```python
from build123d import *

# Parameters (mm, degrees)
EXTRUDE_1_DEPTH           = 18
CHAMFER_1_SIZE            = 5
CHAMFER_2_SIZE            = 5
CUT_EXTRUDE_1_DEPTH       = 8
EXTRUDE_2_REACH           = 696.741
EXTRUDE_2_END_RADIUS      = 240
EXTRUDE_3_DEPTH           = 5
EXTRUDE_4_REACH           = 929.644
EXTRUDE_4_END_RADIUS      = 232
SKETCH_10_R               = 12
CUT_EXTRUDE_7_DEPTH       = 695.872110635
CUT_EXTRUDE_7_DEPTH_BACK  = 695.872110635
SKETCH_16_OUTSIDE_W       = 362.68
SKETCH_16_OUTSIDE_H       = 1204.68
SKETCH_16_OUTSIDE_W_2     = 100
SKETCH_16_OUTSIDE_H_2     = 230
CUT_EXTRUDE_9_DEPTH       = 203.111355445
CUT_EXTRUDE_9_DEPTH_BACK  = 203.111355445
EXTRUDE_5_DEPTH           = 20
CUT_EXTRUDE_10_DEPTH      = 219.63208799
CUT_EXTRUDE_10_DEPTH_BACK = 219.63208799
SKETCH_21_R               = 1.9
EXTRUDE_START             = 15
SKETCH_29_R               = 1.9
EXTRUDE_6_DEPTH           = 15
SKETCH_33_OUTSIDE_W       = 126.318
SKETCH_33_OUTSIDE_H       = 74.662
CUT_EXTRUDE_16_DEPTH      = 40
CUT_EXTRUDE_15_DEPTH      = 41


with BuildPart() as part:
    # Sketch 4 → Loft 1 section 0
    with BuildSketch(Plane(origin=(0, 10, 0), x_dir=(1, 0, 0), z_dir=(0, 1, 0))):
        with BuildLine():
            Line((25, 0), (-25, 0))
            Line((-25, 0), (-25, 630))
            Line((-25, 630), (0, 672.857142857))
            Line((0, 672.857142857), (25, 630))
            Line((25, 630), (25, 0))
        make_face()
    # Sketch 1 → Loft 1 section 1
    with BuildSketch(Plane(origin=(0, 0, 0), x_dir=(1, 0, 0), z_dir=(0, 1, 0))):
        with BuildLine():
            Line((-35, 0), (35, 0))
            Line((35, 0), (35, 630))
            Line((35, 630), (0, 690))
            Line((0, 690), (-35, 630))
            Line((-35, 630), (-35, 0))
        make_face()
    loft_1 = loft()

    # Mirror 1: Loft 1 across plane
    add(loft_1.mirror(Plane.ZX))



with BuildPart() as body_2:
    # Sketch 5 → Extrude 1 (new, symmetric)
    with BuildSketch(Plane(origin=(0, 0, 0), x_dir=(1, 0, 0), z_dir=(0, 1, 0))):
        with BuildLine():
            ThreePointArc((-66.346774613, -65.189169183), (0, -55.5), (66.346774613, -65.189169183))
            ThreePointArc((66.346774613, -65.189169183), (73.061224406, -64.270510235), (76.791165228, -58.612302768))
            ThreePointArc((76.791165228, -58.612302768), (79, -30.5), (76.791165228, -2.387697232))
            ThreePointArc((76.791165228, -2.387697232), (0, -15.004503167), (-76.791165228, -2.387697232))
            ThreePointArc((-76.791165228, -2.387697232), (-79, -30.5), (-76.791165228, -58.612302768))
            ThreePointArc((-76.791165228, -58.612302768), (-73.061224406, -64.270510235), (-66.346774613, -65.189169183))
        make_face()
    extrude(amount=EXTRUDE_1_DEPTH, both=True)

    # Chamfer 1
    chamfer_1_edges = [body_2.edges().sort_by_distance(p)[0] for p in [
        (0, 18, 15.004503167),
        (-79, 18, 30.5),
        (-73.061224406, 18, 64.270510235),
        (0, 18, 55.5),
        (73.061224406, 18, 64.270510235),
        (0, -18, 55.5),
        (-73.061224406, -18, 64.270510235),
        (-79, -18, 30.5),
        (79, -18, 30.5),
        (73.061224406, -18, 64.270510235),
        (79, 18, 30.5),
    ]]
    chamfer(chamfer_1_edges, length=CHAMFER_1_SIZE)

    # Chamfer 2
    chamfer_2_edges = [body_2.edges().sort_by_distance(p)[0] for p in [
        (0, -18, 15.004503167),
    ]]
    chamfer(chamfer_2_edges, length=CHAMFER_2_SIZE)

    # Sketch 6 → Cut-Extrude 1 (cut)
    with BuildSketch(Plane(origin=(0, 18, 0), x_dir=(1, 0, 0), z_dir=(0, 1, 0))):
        with BuildLine():
            ThreePointArc((67.221840199, -55.023712607), (68.932610365, -35.286223394), (68.335500378, -15.483731767))
            ThreePointArc((68.335500378, -15.483731767), (0, -25.004503167), (-68.335500378, -15.483731767))
            ThreePointArc((-68.335500378, -15.483731767), (-68.932610365, -35.286223394), (-67.221840199, -55.023712607))
            ThreePointArc((-67.221840199, -55.023712607), (0, -45.5), (67.221840199, -55.023712607))
        make_face()
    cut_extrude_1 = extrude(amount=-CUT_EXTRUDE_1_DEPTH, mode=Mode.SUBTRACT)

    # Mirror 2: Cut-Extrude 1 across plane
    add(cut_extrude_1.mirror(Plane.ZX), mode=Mode.SUBTRACT)


with BuildPart() as part_1:
    add(part.part)

    add(body_2.part)  # Extrude 2 merges body 2
    # Extrude 2: up to this cylinder (the profile starts inside it)
    extrude_2_end = Plane(origin=(0, 0, -224.995496833), z_dir=(0, -1, 0)) * Cylinder(EXTRUDE_2_END_RADIUS, 1874.482, mode=Mode.PRIVATE)
    # Sketch 7 → Extrude 2 (add, up to the surface)
    with BuildSketch(Plane.XY, mode=Mode.PRIVATE) as extrude_2_sk1:
        Polygon((-25.828427125, 12), (-37.828427125, 0), (-25.828427125, -12), (25.828427125, -12), (37.828427125, 0), (25.828427125, 12), align=None)
    extrude_2_tool1 = extrude(extrude_2_sk1.sketch, amount=EXTRUDE_2_REACH, mode=Mode.PRIVATE) & extrude_2_end
    add(extrude_2_tool1.solids().sort_by_distance((0, 0, 0))[0])

    # Sketch 8 → Extrude 3 (add)
    with BuildSketch(Plane(origin=(0, 0, 0), x_dir=(-1, 0, 0), z_dir=(0, 0, -1))):
        Polygon((25.828427125, 12), (-25.828427125, 12), (-37.828427125, 0), (-25.828427125, -12), (25.828427125, -12), (37.828427125, 0), align=None)
    extrude(amount=EXTRUDE_3_DEPTH)



with BuildPart() as body_2_2:
    # Sketch 9 → Revolve 1 (revolve)
    with BuildSketch(Plane(origin=(0, 0, 0), x_dir=(1, 0, 0), z_dir=(0, 1, 0))):
        Polygon((0, -310), (0, -234), (-12, -234), (-22.5, -256), align=None)
    revolve(axis=Axis((0, 0, -690), (0, 0, 1)))


with BuildPart() as part_2:
    add(part_1.part)

    add(body_2_2.part)  # Extrude 4 merges body 2 2
    # Extrude 4: up to this cylinder (the profile starts inside it)
    extrude_4_end = Plane(origin=(0, 0, 287.5), z_dir=(0, -1, 0)) * Cylinder(EXTRUDE_4_END_RADIUS, 2324.288, mode=Mode.PRIVATE)
    # Sketch 10 → Extrude 4 (add, up to the surface)
    with BuildSketch(Plane(origin=(0, 0, 234), x_dir=(-1, 0, 0), z_dir=(0, 0, -1)), mode=Mode.PRIVATE) as extrude_4_sk1:
        with Locations(Location((0, 0, 0), (0, 0, 90))):
            Circle(SKETCH_10_R)
    extrude_4_tool1 = extrude(extrude_4_sk1.sketch, amount=EXTRUDE_4_REACH, mode=Mode.PRIVATE) & extrude_4_end
    add(extrude_4_tool1.solids().sort_by_distance((0, 0, 234))[0])

    # Sketch 16 outside → Cut-Extrude 7 (cut, two sides: drawn at the far end of the back side and taken through both)
    with BuildSketch(Plane(origin=(0, 0, 0), x_dir=(1, 0, 0), z_dir=(0, 1, 0)).offset(-CUT_EXTRUDE_7_DEPTH_BACK)):
        with Locations((0, 190)):
            Rectangle(SKETCH_16_OUTSIDE_W, SKETCH_16_OUTSIDE_H)
        with Locations((0, 80)):
            Rectangle(SKETCH_16_OUTSIDE_W_2, SKETCH_16_OUTSIDE_H_2, mode=Mode.SUBTRACT)
    extrude(amount=CUT_EXTRUDE_7_DEPTH + CUT_EXTRUDE_7_DEPTH_BACK, mode=Mode.SUBTRACT)

    # Sketch 19 → Cut-Extrude 9 (cut, two sides: drawn at the far end of the back side and taken through both)
    with BuildSketch(Plane(origin=(0, 0, 0), x_dir=(1, 0, 0), z_dir=(0, 1, 0)).offset(-CUT_EXTRUDE_9_DEPTH_BACK)):
        with BuildLine():
            Line((-50, -9.738395054), (-50, -35))
            Line((-50, -35), (50, -35))
            Line((50, -35), (50, -9.738395054))
            ThreePointArc((50, -9.738395054), (0, -15.004503167), (-50, -9.738395054))
        make_face()
    extrude(amount=CUT_EXTRUDE_9_DEPTH + CUT_EXTRUDE_9_DEPTH_BACK, mode=Mode.SUBTRACT)

    # Sketch 20 → Extrude 5 (add)
    with BuildSketch(Plane.XY):
        Polygon((-25.828427125, 12), (-37.828427125, 0), (-25.828427125, -12), (25.828427125, -12), (37.828427125, 0), (25.828427125, 12), align=None)
    extrude(amount=EXTRUDE_5_DEPTH)

    # Sketch 21 → Cut-Extrude 10 (cut, two sides: drawn at the far end of the back side and taken through both)
    with BuildSketch(Plane.XY.offset(20).offset(-CUT_EXTRUDE_10_DEPTH_BACK)):
        Circle(SKETCH_21_R)
    extrude(amount=CUT_EXTRUDE_10_DEPTH + CUT_EXTRUDE_10_DEPTH_BACK, mode=Mode.SUBTRACT)

    # Sketch 29 → Extrude 6 (add)
    with BuildSketch(Plane.XY.offset(20).offset(EXTRUDE_START)):
        Polygon((25.828427125, 12), (-25.828427125, 12), (-37.828427125, 0), (-25.828427125, -12), (25.828427125, -12), (37.828427125, 0), align=None)
        Circle(SKETCH_29_R, mode=Mode.SUBTRACT)
    extrude(amount=-EXTRUDE_6_DEPTH)

    # Sketch 33 outside → Cut-Extrude 16 (cut)
    with BuildSketch(Plane.XY.offset(35)):
        Rectangle(SKETCH_33_OUTSIDE_W, SKETCH_33_OUTSIDE_H)
        Polygon((30.757359313, 0), (23.757359313, 7), (-23.757359313, 7), (-30.757359313, 0), (-23.757359313, -7), (23.757359313, -7), align=None, mode=Mode.SUBTRACT)
    extrude(amount=-CUT_EXTRUDE_16_DEPTH, mode=Mode.SUBTRACT)

    # Sketch 31 → Cut-Extrude 15 (cut)
    with BuildSketch(Plane(origin=(0, 0, -195), x_dir=(-1, 0, 0), z_dir=(0, 0, -1))):
        Polygon((-28.211774901, 0), (-23.011774901, -5.2), (23.011774901, -5.2), (28.211774901, 0), (23.011774901, 5.2), (-23.011774901, 5.2), align=None)
    extrude(amount=-CUT_EXTRUDE_15_DEPTH, mode=Mode.SUBTRACT)


solid = part_2.part
```
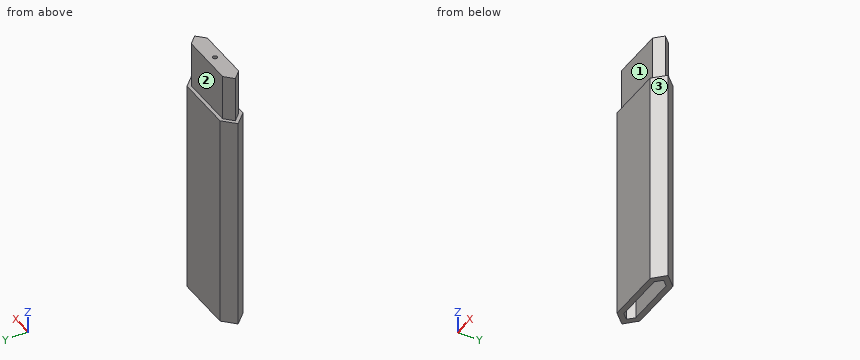
The model under review builds one solid part; all positions refer to its coordinate system, in mm. Face numbers are marked on the shaded views. A direction names the side the tool comes from. Give positions to 0.01 mm unless a question says otherwise; leave off trailing zeros. Write each loop counter-clockwise with the first axis right and the second up, starting at its lowest first coordinate (ties: lowest second). Pieces come first, ordered by that corner, then holes.
(1) Consider section B-B, the plane z = 14.5. Give the boundary of the cut face in (x, y).
(2) Consider section D-D, the plane z = -41. Give the boundary of the cut face in (x, y), and give its area (3 significant figures).
(3) Consider section C-C, the plane x = 5.5. Give the boundary of the cut face in (y, z).
(4) For P1, Ø4, axis at y = -1, z = -58.5, coming from the -X side; P2, Ø12, axis at x = -2.5, z = 17.5, coming from the +Y side; P3, Ø5, axis at x = 0, y = 0, coming from the -Z side, all flat-tipped, find the tip position at first contact; note any pin that passes through.
(5) Tool access review of the marked faces 1, 2 and 3: name each direction out of +Z, -Z, +X, -X, +Y, -Y from which nothing blocks a thin tool from reaching the whole face with its end or side.
(6) Consider section A-A, the plane z = -171. Give the boundary of the cut face in (x, y), and give its area (3 significant figures).
(7) To check wall thickness, follow L1, parallel to Y at x = 0, z = 27; L2, parallel to X at y = 0, z = 23; L3, parallel to Y at x = 0, z = -16.5. State the ranges of each line that lie inside material, in increasing order.
Returned:
1. outline: (-30.76, 0) - (-23.76, -7) - (23.76, -7) - (30.76, 0) - (23.76, 7) - (-23.76, 7) - close; hole circle Ø3.8 at (0, 0)
2. outline: (-35, 0) - (-25, -10) - (25, -10) - (35, 0) - (25, 10) - (-25, 10) - close; hole circle Ø3.8 at (0, 0)
2. area: 1,190 mm2
3. outline: (-10, -195) - (-5.2, -195) - (-5.2, -154) - (5.2, -154) - (5.2, -195) - (10, -195) - (10, -5) - (7, -5) - (7, 35) - (-7, 35) - (-7, -5) - (-10, -5) - close
4. P1: stops at x = -35
4. P2: stops at y = 7
4. P3: stops at z = -154
5. face 1: +Z, +X, -X, -Y
5. face 2: +Z, +X, -X, +Y
5. face 3: +Z, -Z, +X, -Y
6. outline: (-35, 0) - (-25, -10) - (25, -10) - (35, 0) - (25, 10) - (-25, 10) - close; hole (-28.21, 0) - (-23.01, -5.2) - (23.01, -5.2) - (28.21, 0) - (23.01, 5.2) - (-23.01, 5.2) - close
6. area: 667 mm2
7. L1: y = -7 to -1.9, 1.9 to 7
7. L2: x = -30.76 to -1.9, 1.9 to 30.76
7. L3: y = -10 to -1.9, 1.9 to 10
